Model file for the job. Use its own axes, mm. A direction names the side the tool comes from. Round coordinates to 2 decimals unless told otherwise and drop trailing zeros. Loops run counter-clockwise (first coordinate to the right, second up) from the corner with the lowest first, then second, coordinate; pieces in that order, holes last. Notation, with made-up numbers: (48, -25.5) -> (60, -25.5) arc R28 cw to (60, -7.5) -> close; hole circle Ø11 at (75, 16). An arc over 180 degrees is marked (long way). Use a Markdown table: item, result.
from build123d import *

# Parameters (mm, degrees)
BOSS_EXTRUDE1_DEPTH                                 = 20
SKETCH1_3_W                                         = 45
SKETCH1_3_H                                         = 45
CUT_EXTRUDE2_DEPTH                                  = 5
CBORE_FOR_M8_HEX_SOCKET_HEAD_CAP_SCREW1_D           = 9
CBORE_FOR_M8_HEX_SOCKET_HEAD_CAP_SCREW1_DEPTH       = 23
CBORE_FOR_M8_HEX_SOCKET_HEAD_CAP_SCREW1_CBORE_D     = 15
CBORE_FOR_M8_HEX_SOCKET_HEAD_CAP_SCREW1_CBORE_DEPTH = 8.6
CBORE_FOR_M8_HEX_SOCKET_HEAD_CAP_SCREW1_TIP         = 2.703872786
FILLET2_R                                           = 2.5
SKETCH4_R                                           = 11
CUT_EXTRUDE3_DEPTH                                  = 6
SKETCH5_R                                           = 14
CUT_EXTRUDE4_DEPTH                                  = 1
CUT_EXTRUDE4_DEPTH_BACK                             = 15
CHAMFER1_SIZE                                       = 0.5
CBORE_FOR_M5_HEX_SOCKET_HEAD_CAP_SCREW1_D           = 5.5
CBORE_FOR_M5_HEX_SOCKET_HEAD_CAP_SCREW1_CBORE_D     = 10
CBORE_FOR_M5_HEX_SOCKET_HEAD_CAP_SCREW1_CBORE_DEPTH = 5.4


with BuildPart() as part:
    # Sketch1 → Boss-Extrude1 (new body)
    with BuildSketch(Plane.XY):
        with BuildLine():
            Line((-52.5, 17), (-43.072613109, 17))
            ThreePointArc((-43.072613109, 17), (-35.337121021, 18.746933761), (-29.103116965, 23.648648649))
            ThreePointArc((-29.103116965, 23.648648649), (37.5, 0), (-29.103116965, -23.648648649))
            ThreePointArc((-29.103116965, -23.648648649), (-35.337121021, -18.746933761), (-43.072613109, -17))
            Line((-43.072613109, -17), (-52.5, -17))
            ThreePointArc((-52.5, -17), (-69.5, 0), (-52.5, 17))
        make_face()
    extrude(amount=BOSS_EXTRUDE1_DEPTH)

    # Sketch1<3> → Cut-Extrude2 (cut)
    with BuildSketch(Plane.XY):
        Rectangle(SKETCH1_3_W, SKETCH1_3_H)
    extrude(amount=CUT_EXTRUDE2_DEPTH, mode=Mode.SUBTRACT)

    # CBORE for M8 Hex Socket Head Cap Screw1
    with Locations(Plane.XY.offset(20)):
        with Locations((0, 0)):
            CounterBoreHole(CBORE_FOR_M8_HEX_SOCKET_HEAD_CAP_SCREW1_D / 2, CBORE_FOR_M8_HEX_SOCKET_HEAD_CAP_SCREW1_CBORE_D / 2, CBORE_FOR_M8_HEX_SOCKET_HEAD_CAP_SCREW1_CBORE_DEPTH, depth=CBORE_FOR_M8_HEX_SOCKET_HEAD_CAP_SCREW1_DEPTH)
            with Locations((0, 0, -(CBORE_FOR_M8_HEX_SOCKET_HEAD_CAP_SCREW1_DEPTH + CBORE_FOR_M8_HEX_SOCKET_HEAD_CAP_SCREW1_TIP / 2))):  # 118° drill point
                Cone(0, CBORE_FOR_M8_HEX_SOCKET_HEAD_CAP_SCREW1_D / 2, CBORE_FOR_M8_HEX_SOCKET_HEAD_CAP_SCREW1_TIP, mode=Mode.SUBTRACT)

    # Fillet2
    fillet2_edges = [part.edges().sort_by_distance(p)[0] for p in [
        (-22.5, 22.5, 2.5),
        (22.5, 22.5, 2.5),
        (22.5, -22.5, 2.5),
        (-22.5, -22.5, 2.5),
    ]]
    fillet(fillet2_edges, radius=FILLET2_R)

    # Sketch4 → Cut-Extrude3 (cut)
    with BuildSketch(Plane(origin=(0, 0, 0), x_dir=(-1, 0, 0), z_dir=(0, 0, -1))):
        with Locations((52.5, 0)):
            Circle(SKETCH4_R)
    extrude(amount=-CUT_EXTRUDE3_DEPTH, mode=Mode.SUBTRACT)

    # Sketch5 → Cut-Extrude4 (cut, two sides)
    with BuildSketch(Plane(origin=(0, 0, 6), x_dir=(-1, 0, 0), z_dir=(0, 0, -1))) as cut_extrude4_sk:
        with Locations((52.5, 0)):
            Circle(SKETCH5_R)
    extrude(amount=CUT_EXTRUDE4_DEPTH, mode=Mode.SUBTRACT)
    extrude(cut_extrude4_sk.sketch, amount=-CUT_EXTRUDE4_DEPTH_BACK, mode=Mode.SUBTRACT)

    # Chamfer1
    chamfer1_edges = [part.edges().sort_by_distance(p)[0] for p in [
        (-47.786306554, 17, 20),
        (-69.5, 0, 20),
        (-47.786306554, -17, 20),
        (-35.337121021, -18.746933761, 20),
        (-7.5, 0, 20),
        (37.5, 0, 20),
        (22.5, 0, 0),
        (0, 22.5, 0),
        (0, -22.5, 0),
        (-22.5, 0, 0),
        (21.767766953, 21.767766953, 0),
        (21.767766953, -21.767766953, 0),
        (-21.767766953, -21.767766953, 0),
        (-21.767766953, 21.767766953, 0),
        (-35.337121021, -18.746933761, 0),
        (-41.5, 0, 0),
        (-47.786306554, -17, 0),
        (-38.5, 0, 20),
        (-69.5, 0, 0),
        (-35.337121021, 18.746933761, 20),
        (-47.786306554, 17, 0),
        (-35.337121021, 18.746933761, 0),
        (37.5, 0, 0),
    ]]
    chamfer(chamfer1_edges, length=CHAMFER1_SIZE)

    # CBORE for M5 Hex Socket Head Cap Screw1 (through all)
    with Locations(Plane(origin=(0, 0, 0), x_dir=(-1, 0, 0), z_dir=(0, 0, -1))):
        with Locations((0, 30), (-30, 0), (0, -30), (30, 0)):
            CounterBoreHole(CBORE_FOR_M5_HEX_SOCKET_HEAD_CAP_SCREW1_D / 2, CBORE_FOR_M5_HEX_SOCKET_HEAD_CAP_SCREW1_CBORE_D / 2, CBORE_FOR_M5_HEX_SOCKET_HEAD_CAP_SCREW1_CBORE_DEPTH)


solid = part.part
Q1. Band-saw the part on D-D, the plane z = 17.75. Give the cut face in (x, y), plus the area to 3 significant figures.
Results list:
| item | result |
|---|---|
| outline | (-52.5, -17) -> (-43.07, -17) arc R18 cw to (-29.1, -23.65) arc R37.5 ccw (long way) to (-29.1, 23.65) arc R18 cw to (-43.07, 17) -> (-52.5, 17) arc R17 ccw to start; hole circle Ø28 at (-52.5, 0); hole circle Ø5.5 at (-30, 0); hole circle Ø15 at (0, 0); hole circle Ø5.5 at (0, -30); hole circle Ø5.5 at (0, 30); hole circle Ø5.5 at (30, 0) |
| area | 4,560 mm² |
Q2. Pull direction Y, two halves, no side cores. Call faces 1 (the face through (-27, -8, 0)), 2 (the face through (-0.358, -27.273, 12.802)), 3 (the face through (-35.44, 18.7, 9.87)): released by +Y, released by -Y, zero draft, split by the parting line, or undercut.
Results list:
| item | result |
|---|---|
| face 1 | zero draft |
| face 2 | undercut |
| face 3 | released by +Y |
Q3. Drill centre lines: L1, parallel to Y at x = 0, z = 9; L2, parallel to Z at x = -42.5, y = -6.5; L3, parallel to Y at x = -1.5, z = 2.5. Where is each one in solid material? Low to high. Write a range as from..to.
Results list:
| item | result |
|---|---|
| L1 | y = -37.5..-32.75, -27.25..-4.5, 4.5..27.25, 32.75..37.5 |
| L2 | z = 0..5 |
| L3 | y = -37.47..-34.77, -25.23..-22.5, 22.5..25.23, 34.77..37.47 |
Q4. Band-saw the part on B-B, the plane x = 0. Give the number of separate pieces and of enclosed holes in the cut face, plus the area to 3 significant figures.
Results list:
| item | result |
|---|---|
| separate pieces | 4 |
| enclosed holes | 0 |
| area | 819 mm² |
Q5. Flat gauge pins, fed straight in: pin 1 (17 mm diameter, centred on x = -52.5, y = 0, fed in from +Z); pin 2 (3 mm diameter, centred on x = -1.5, y = 28, fed in from -Z); pin 3 (1.5 mm diameter, centred on y = 27, z = 8, fed in from -X); pin 4 (12 mm diameter, centred on y = 27.5, z = 6.5, fed in from -X). Where does each tip first touch, or does it go through?
Results list:
| item | result |
|---|---|
| pin 1 | passes through |
| pin 2 | stops at z = 5.4 |
| pin 3 | stops at x = -26.78 |
| pin 4 | stops at x = -31.17 |
Q6. Band-saw the part on A-A, the plane z = 3.75. Give the cut face in (x, y), plus the area to 3 significant figures.
Results list:
| item | result |
|---|---|
| outline | (-52.5, -17) -> (-43.07, -17) arc R18 cw to (-29.1, -23.65) arc R37.5 ccw (long way) to (-29.1, 23.65) arc R18 cw to (-43.07, 17) -> (-52.5, 17) arc R17 ccw to start; hole circle Ø22 at (-52.5, 0); hole circle Ø10 at (-30, 0); hole (-22.5, -20) arc R2.5 ccw to (-20, -22.5) -> (20, -22.5) arc R2.5 ccw to (22.5, -20) -> (22.5, 20) arc R2.5 ccw to (20, 22.5) -> (-20, 22.5) arc R2.5 ccw to (-22.5, 20) -> close; hole circle Ø10 at (0, -30); hole circle Ø10 at (0, 30); hole circle Ø10 at (30, 0) |
| area | 2,740 mm² |
Q7. Tool access for faces 4 (the face through (-58.7, -9.3, 5)), 5 (the face through (-48, 17, 10)), 6 (the face through (-48, -17, 10)), 7 (the face through (22.5, 0, 3)): list every direction of +Z, -Z, +X, -X, +Y, -Y with a clear straight run to the whole face (end or side of a thin tool).
Results list:
| item | result |
|---|---|
| face 4 | +Z |
| face 5 | +Z, -Z, -X, +Y |
| face 6 | +Z, -Z, -X, -Y |
| face 7 | -Z |
